Read the model definition and answer for the solid it produces. Units are mm, in the model's axes. Face numbers are marked on the shaded views. A direction names the side the tool comes from. Coordinates: 2 decimals unless noted, no trailing zeros. Loops run counter-clockwise (first coordinate to the right, second up) from the corner with the lowest first, then second, coordinate; pieces in that order, holes last. Notation, with made-up numbers: (20, 22) - (40, 22) arc R22 cw to (40, 41) - close; hole circle Ø10 at (57, 49.25). An arc over 180 degrees is marked (long way). Use one line per item in the form item = value.
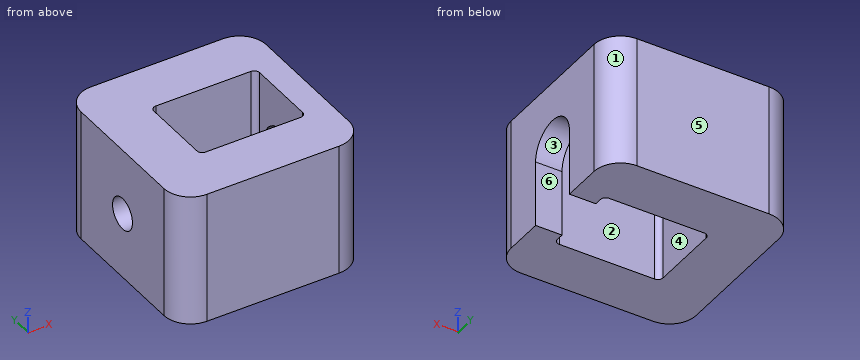
from build123d import *

# Parameters (mm, degrees)
F0_W     = 10
F0_H     = 15
F0_W_2   = 5
F0_H_2   = 10.2
F1_DEPTH = 25
F3_DEPTH = 15
F4_R     = 3
F5_DEPTH = 25
F6_R     = 1
F7_R     = 5


with BuildPart() as f1:
    # F0 (on Top) → F1 (new body)
    with BuildSketch(Plane.XY):
        Polygon((15, -17.5), (15, -7.5), (-5, -7.5), (-15, -7.5), (-15, -17.5), align=None)
        with Locations((-10, 0)):
            Rectangle(F0_W, F0_H)
        Polygon((-15, 7.5), (-5, 7.5), (15, 7.5), (15, 17.5), (-15, 17.5), align=None)
        Polygon((15, 7.5), (15, 5.1), (20, 5.1), (20, 17.5), (15, 17.5), align=None)
        with Locations((17.5, 0)):
            Rectangle(F0_W_2, F0_H_2)
        Polygon((15, -5.1), (15, -7.5), (15, -17.5), (20, -17.5), (20, -5.1), align=None)
    extrude(amount=F1_DEPTH)

    # F2 (on face) → F3 (cut)
    with BuildSketch(Plane.YZ.offset(20)):
        with BuildLine():
            ThreePointArc((-5.1, 12.5), (0, 7.4), (5.1, 12.5))
            ThreePointArc((5.1, 12.5), (0, 17.6), (-5.1, 12.5))
        make_face()
        with BuildLine():
            Line((5.1, 0), (5.1, 12.5))
            ThreePointArc((5.1, 12.5), (0, 7.4), (-5.1, 12.5))
            Line((-5.1, 12.5), (-5.1, 0))
            Line((-5.1, 0), (5.1, 0))
        make_face()
    extrude(amount=-F3_DEPTH, mode=Mode.SUBTRACT)

    # F4 (on face) → F5 (cut)
    with BuildSketch(Plane(origin=(-15, 0, 0), x_dir=(0, -1, 0), z_dir=(-1, 0, 0))):
        with Locations((0, 12.5)):
            Circle(F4_R)
    extrude(amount=-F5_DEPTH, mode=Mode.SUBTRACT)

    # F6
    f6_edges = [f1.edges().sort_by_distance(p)[0] for p in [
        (15, -7.5, 12.5),
        (15, 7.5, 12.5),
        (-5, -7.5, 12.5),
        (-5, 7.5, 12.5),
    ]]
    fillet(f6_edges, radius=F6_R)

    # F7
    f7_edges = [f1.edges().sort_by_distance(p)[0] for p in [
        (20, 17.5, 12.5),
        (20, -17.5, 12.5),
        (-15, -17.5, 12.5),
        (-15, 17.5, 12.5),
    ]]
    fillet(f7_edges, radius=F7_R)


solid = f1.part
Item 1: Which of the six approach directions +Z, -Z, +X, -X, +Y, -Y give full straight-line access (tool end or side, diameter ignored) to the marked faces 4, 5 and 6?
Results below:
face_4 = +Z, -Z
face_5 = +Z, -Z, +X, -X, +Y
face_6 = -Z, +X
Item 2: The part is cut by section B-B on x = 8.5. Give the vertices of the cut face in (y, z), plus the area to 3 significant figures.
Results below:
outline = (-17.5, 0) - (-7.5, 0) - (-7.5, 25) - (-17.5, 25) - close; (7.5, 0) - (17.5, 0) - (17.5, 25) - (7.5, 25) - close
area = 500 mm²
Item 3: The part is cut by section D-D on y = 0. Give the vertices of the cut face in (x, z).
Results below:
outline = (-15, 0) - (-5, 0) - (-5, 9.5) - (-15, 9.5) - close; (-15, 15.5) - (-5, 15.5) - (-5, 25) - (-15, 25) - close; (15, 17.6) - (20, 17.6) - (20, 25) - (15, 25) - close
Item 4: For a pull along X with two mould halves and no side action, classify the marked faces 1, 2 and 3 as +X half, -X half, draft (parallel to the pull), parting line (faces both ways), or undercut.
Results below:
face_1 = +X half
face_2 = undercut
face_3 = draft
Item 5: Each of these flat-tipped pins is pushed along its axis until it touches: P1, Ø14.5, axis at y = -2.5, z = 8, coming from the +X side; P2, Ø1.5, axis at x = 16.5, z = 6, coming from the +Y side; P3, Ø3, axis at y = -3, z = 3, coming from the +X side; P4, Ø2.5, axis at x = 18.5, z = 5, coming from the -Y side. Where does it stop, or does it pass through?
Results below:
P1 = 20
P2 = 17.44
P3 = -5
P4 = -16.97
Item 6: Find the intervals of material crossed by L1, parallel to Z at x = -10, y = 0; L2, parallel to X at y = -5, z = 17.5; L3, parallel to Y at x = 2, z = 5.25, in increasing order.
Results below:
L1 = 0 to 9.5, 15.5 to 25
L2 = -15 to -5, 15 to 20
L3 = -17.5 to -7.5, 7.5 to 17.5
Item 7: The part is cut by section C-C on y = -4.5. Give the vertices of the cut face in (x, z), plus the area to 4 significant figures.
Results below:
outline = (-15, 0) - (-5, 0) - (-5, 25) - (-15, 25) - close; (15, 14.9) - (20, 14.9) - (20, 25) - (15, 25) - close
area = 300.5 mm²
Item 8: The part is cut by section A-A on z = 21.25. Give the vertices of the cut face in (x, y), plus the area to 3 significant figures.
Results below:
outline = (-15, -12.5) arc R5 ccw to (-10, -17.5) - (15, -17.5) arc R5 ccw to (20, -12.5) - (20, 12.5) arc R5 ccw to (15, 17.5) - (-10, 17.5) arc R5 ccw to (-15, 12.5) - close; hole (-5, -6.5) arc R1 ccw to (-4, -7.5) - (14, -7.5) arc R1 ccw to (15, -6.5) - (15, 6.5) arc R1 ccw to (14, 7.5) - (-4, 7.5) arc R1 ccw to (-5, 6.5) - close
area = 904 mm²
